Can you work these out from the model? Positions are in its coordinate system, mm. A direction names the side the tool comes from. Round coordinates to 2 decimals unless told otherwise and drop trailing zeros. Loops run counter-clockwise (first coordinate to the right, second up) from the corner with the lowest first, then second, coordinate; pieces in that order, holes last. Notation, with made-up numbers: M -39.75,-1.75 L -25.75,-1.75 A16 cw -25.75,9.25 Z; hole C 45,-19 d4. An arc over 180 degrees is marked long. Answer as CSV lines item,"result".
from build123d import *

# Parameters (mm, degrees)
SKETCH1_R                = 7.5
BOSS_EXTRUDE1_DEPTH      = 12
SKETCH3_R                = 30
BOSS_EXTRUDE2_DEPTH      = 68
HOLE1_D                  = 30
HOLE1_DEPTH              = 80
HOLE1_CBORE_D            = 40
HOLE1_CBORE_DEPTH        = 16
HOLE1_TIP                = 9.012909285
BOSS_EXTRUDE3_REACH      = 135.884
BOSS_EXTRUDE3_END_RADIUS = 30
CUT_EXTRUDE1_REACH       = 135.884
CUT_EXTRUDE1_END_RADIUS  = 15
SKETCH11_R               = 8


with BuildPart() as part:
    # Sketch1 → Boss-Extrude1 (new body)
    with BuildSketch(Plane(origin=(0, 0, 0), x_dir=(1, 0, 0), z_dir=(0, 1, 0))):
        with BuildLine():
            Line((-50, 35), (-50, -35))
            ThreePointArc((-50, -35), (-45.606601718, -45.606601718), (-35, -50))
            Line((-35, -50), (68, -50))
            ThreePointArc((68, -50), (73.740251485, -48.858192988), (78.606601718, -45.606601718))
            Line((78.606601718, -45.606601718), (105.606601718, -18.606601718))
            ThreePointArc((105.606601718, -18.606601718), (109.871672921, -6.042107117), (102.5, 4.990381057))
            Line((102.5, 4.990381057), (28.021815275, 47.990381057))
            ThreePointArc((28.021815275, 47.990381057), (24.404100951, 49.488887394), (20.521815275, 50))
            Line((20.521815275, 50), (-35, 50))
            ThreePointArc((-35, 50), (-45.606601718, 45.606601718), (-50, 35))
        make_face()
        with Locations(Location((95, -8, 0), (0, 0, 270))):
            Circle(SKETCH1_R, mode=Mode.SUBTRACT)
        with Locations(Location((-35, 35, 0), (0, 0, 270))):
            Circle(SKETCH1_R, mode=Mode.SUBTRACT)
        with Locations(Location((-35, -35, 0), (0, 0, 270))):
            Circle(SKETCH1_R, mode=Mode.SUBTRACT)
    extrude(amount=BOSS_EXTRUDE1_DEPTH)

    # Sketch3 → Boss-Extrude2 (add)
    with BuildSketch(Plane(origin=(0, 12, 0), x_dir=(1, 0, 0), z_dir=(0, 1, 0))):
        with Locations(Location((0, 0, 0), (0, 0, 270))):
            Circle(SKETCH3_R)
    extrude(amount=BOSS_EXTRUDE2_DEPTH)

    # Hole1
    with Locations(Plane(origin=(0, 80, 0), x_dir=(1, 0, 0), z_dir=(0, 1, 0))):
        with Locations((0, 0)):
            CounterBoreHole(HOLE1_D / 2, HOLE1_CBORE_D / 2, HOLE1_CBORE_DEPTH, depth=HOLE1_DEPTH)
            with Locations((0, 0, -(HOLE1_DEPTH + HOLE1_TIP / 2))):  # 118° drill point
                Cone(0, HOLE1_D / 2, HOLE1_TIP, mode=Mode.SUBTRACT)

    # Boss-Extrude3: up to this cylinder (the profile starts outside it)
    boss_extrude3_end = Plane(origin=(0, 33.024623, 0), z_dir=(0, -1, 0)) * Cylinder(BOSS_EXTRUDE3_END_RADIUS, 332.768, mode=Mode.PRIVATE)
    # Sketch10 → Boss-Extrude3 (add, up to the surface)
    with BuildSketch(Plane(origin=(45, 0, 0), x_dir=(0, 0, -1), z_dir=(1, 0, 0)), mode=Mode.PRIVATE) as boss_extrude3_sk1:
        with BuildLine():
            Line((-15, 42), (-15, 12))
            Line((-15, 12), (15, 12))
            Line((15, 12), (15, 42))
            ThreePointArc((15, 42), (0, 57), (-15, 42))
        make_face()
    boss_extrude3_tool1 = extrude(boss_extrude3_sk1.sketch, amount=-BOSS_EXTRUDE3_REACH, mode=Mode.PRIVATE) - boss_extrude3_end
    add(boss_extrude3_tool1.solids().sort_by_distance((45, 33.024623, 0))[0])

    # Cut-Extrude1: up to this cylinder (the profile starts outside it)
    cut_extrude1_end = Plane(origin=(0, 42, 0), z_dir=(0, 1, 0)) * Cylinder(CUT_EXTRUDE1_END_RADIUS, 302.768, mode=Mode.PRIVATE)
    # Sketch11 → Cut-Extrude1 (cut, up to the surface)
    with BuildSketch(Plane(origin=(45, 0, 0), x_dir=(0, 0, -1), z_dir=(1, 0, 0)), mode=Mode.PRIVATE) as cut_extrude1_sk1:
        with Locations((0, 42)):
            Circle(SKETCH11_R)
    cut_extrude1_tool1 = extrude(cut_extrude1_sk1.sketch, amount=-CUT_EXTRUDE1_REACH, mode=Mode.PRIVATE) - cut_extrude1_end
    add(cut_extrude1_tool1.solids().sort_by_distance((45, 42, 0))[0], mode=Mode.SUBTRACT)


solid = part.part
Item 1: If we section it at B-B on y = 29: Write out the boundary of the cut face in (x, z), then the cut area to 3 significant figures.
Output:
outline,"M 25.98,-15 L 45,-15 L 45,15 L 25.98,15 A30 ccw long Z; hole C 0,0 d30"
area,"2,610 mm2"
Item 2: We'd pull the mould along X, two halves only. Please class faces 6 (the face through (24.457, 5.916, -49.475)), 7 (the face through (-45.72, 5.92, 45.49)), 8 (the face through (29.07, 44.4, -7.63)), 9 (the face through (-42.32, 5.92, 33.37)): released by +X, released by -X, zero draft, split by the parting line, or undercut.
Output:
face 6,"released by +X"
face 7,"released by -X"
face 8,"zero draft"
face 9,"undercut"
Item 3: If I drill on line 1 along Z through (x, y) = (34, 42); line 2 along Y through (x, z) = (-15.5, -0.5); line 3 along X through (y, z) = (14, -26), over which ranges is the centre line in solid material (lowest first)? Write a range as from..to.
Output:
line 1,"z = -15..-8, 8..15"
line 2,"y = 0..64"
line 3,"x = -14.97..14.97"
Item 4: If we section it at C-C on z = -23: Write out the boundary of the cut face in (x, y).
Output:
outline,"M -50,0 L 71.31,0 L 71.31,12 L 19.26,12 L 19.26,80 L -19.26,80 L -19.26,12 L -50,12 Z"
Item 5: Will these pins go through, and if not, where does the flat tip stop? pin 1 (4 mm diameter, centred on x = 64, z = -14, fed in from +Y); pin 2 (21 mm diameter, centred on x = 34, y = 32.5, fed in from -Z); pin 3 (24 mm diameter, centred on y = 42, z = 7.5, fed in from +X).
Output:
pin 1,"stops at y = 12"
pin 2,"stops at z = -18.65"
pin 3,"stops at x = 45"
Item 6: If we section it at D-D on x = 95: Write out the boundary of the cut face in (y, z).
Output:
outline,"M 0,-9.32 L 12,-9.32 L 12,0.5 L 0,0.5 Z; M 0,15.5 L 12,15.5 L 12,29.21 L 0,29.21 Z"
Item 7: If we section it at A-A on x = 0: Write out the boundary of the cut face in (y, z).
Output:
outline,"M 0,-50 L 12,-50 L 12,-30 L 80,-30 L 80,-20 L 64,-20 L 64,-15 L 0,-15 Z; M 0,15 L 64,15 L 64,20 L 80,20 L 80,30 L 12,30 L 12,50 L 0,50 Z"
Item 8: On a 3-axis mill with a long thin cutter (end or side, diameter ignored), from which of +Z, -Z, +X, -X, +Y, -Y can I reach the whole of each face in a straight line? I mean faces 1 (the face through (36, 27, -15)), 2 (the face through (65.78, 5.92, -26.19)), 3 (the face through (45, 30, 0)), 4 (the face through (3, 64, -15)), 5 (the face through (36, 27, 15)). Say none if no direction works.
Output:
face 1,"-Z, +X, +Y"
face 2,"-Z, +X, +Y, -Y"
face 3,"+Z, -Z, +X, +Y"
face 4,"+Y"
face 5,"+Z, +X, +Y"
